Could you check a few things on this drawing? It's one solid part, dimensions in mm from its lowest x, y, z. A direction names the side the tool comes from. Round coordinates to 2 decimals unless told otherwise and drop trailing zeros. Loops run counter-clockwise (first coordinate to the right, second up) from the corner with the lowest first, then second, coordinate; pieces in that order, holes last. Notation, with made-up numbers: M 59.25,16 L 112.25,16 A6 ccw 112.25,27 Z; hole C 2,-5 d6. An arc over 180 degrees is marked long. Write item = value, one per line. Start each with the question number.
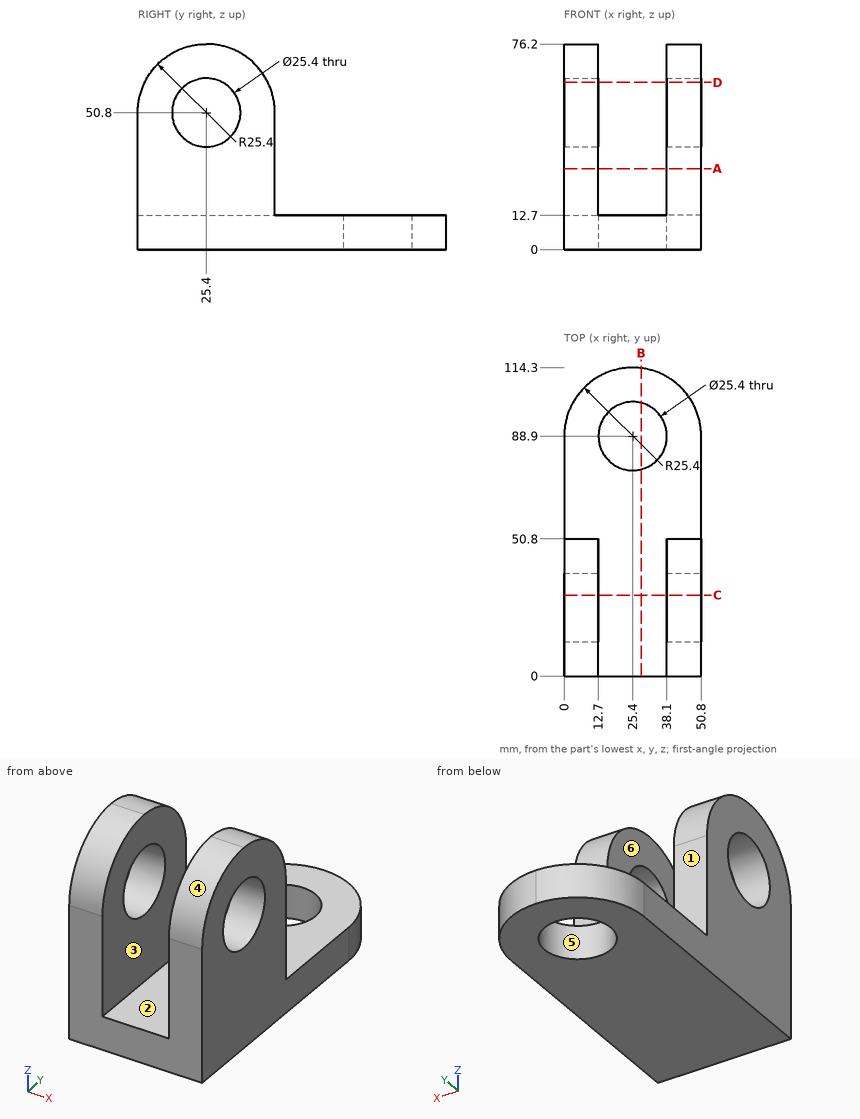
Item 1: For the marked faces 1, 2 and 3, which set-ups out of +Z, -Z, +X, -X, +Y, -Y let a thin tool reach every point of the face, with its end or its side?
Item 2: I want a section at A-A, the plane z = 30. List the corners of the cut face in (x, y) for me.
Item 3: Please list where these lines run through material, in increasing order: line 1 (Z direction, x = 41, y = 25); line 2 (Z direction, x = 26.5, y = 30); line 3 (X direction, y = 26, z = 28.5). Write a range as [from, to].
Item 4: We'd pull the mould along Y, two halves only. Please class the marked faces 4, 5 and 6: released by +Y, released by -Y, zero draft, split by the parting line, or undercut.
Item 5: I want a section at C-C, the plane y = 30. List the corners of the cut face in (x, z) for me, then the cut area to 3 significant figures.
Item 6: I want a section at D-D, the plane z = 62. List the corners of the cut face in (x, y) for me, then the cut area to 3 significant figures.
Item 7: Will these pins go through, and if not, where does the flat tip stop? pin 1 Ø4 at (x, z) = (43, 27.5) entering from +Y; pin 2 Ø15 at (x, y) = (25.5, 33) entering from +Z; pin 3 Ø1.5 at (x, z) = (5, 63.5) entering from -Y.
Item 8: I want a section at B-B, the plane x = 28.5. List the corners of the cut face in (y, z) for me, then the cut area to 3 significant figures.
Worked out:
q1.face_1 = +Z, +X, -X, +Y
q1.face_2 = +Z, +Y
q1.face_3 = +Z, +Y, -Y
q2.outline = M 0,0 L 12.7,0 L 12.7,50.8 L 0,50.8 Z; M 38.1,0 L 50.8,0 L 50.8,50.8 L 38.1,50.8 Z
q3.line_1 = [0, 38.11], [63.49, 76.2]
q3.line_2 = [0, 12.7]
q3.line_3 = [0, 12.7], [38.1, 50.8]
q4.face_4 = released by -Y
q4.face_5 = undercut
q4.face_6 = zero draft
q5.outline = M 0,0 L 50.8,0 L 50.8,38.96 L 38.1,38.96 L 38.1,12.7 L 12.7,12.7 L 12.7,38.96 L 0,38.96 Z; M 0,62.64 L 12.7,62.64 L 12.7,75.78 L 0,75.78 Z; M 38.1,62.64 L 50.8,62.64 L 50.8,75.78 L 38.1,75.78 Z
q5.area = 1,650 mm2
q6.outline = M 0,2.6 L 12.7,2.6 L 12.7,19.41 L 0,19.41 Z; M 0,31.39 L 12.7,31.39 L 12.7,48.2 L 0,48.2 Z; M 38.1,2.6 L 50.8,2.6 L 50.8,19.41 L 38.1,19.41 Z; M 38.1,31.39 L 50.8,31.39 L 50.8,48.2 L 38.1,48.2 Z
q6.area = 854 mm2
q7.pin_1 = 50.8
q7.pin_2 = 12.7
q7.pin_3 = 2.99
q8.outline = M 0,0 L 76.58,0 L 76.58,12.7 L 0,12.7 Z; M 101.22,0 L 114.11,0 L 114.11,12.7 L 101.22,12.7 Z
q8.area = 1,140 mm2
